Could you check a few things on this model? Use its own coordinates, in mm. Round coordinates to 2 decimals unless told otherwise and drop trailing zeros. Write each loop counter-clockwise with the first axis right and the second up, starting at its lowest first coordinate (ties: lowest second). Pieces come first, ordered by that corner, then holes. Notation, with made-up numbers: (32, -31) -> (49, -31) arc R18 cw to (49, -5) -> close; hole circle Ø8 at (18, 12). An arc over 180 degrees is marked (long way). Answer in a Markdown table with one row per item.
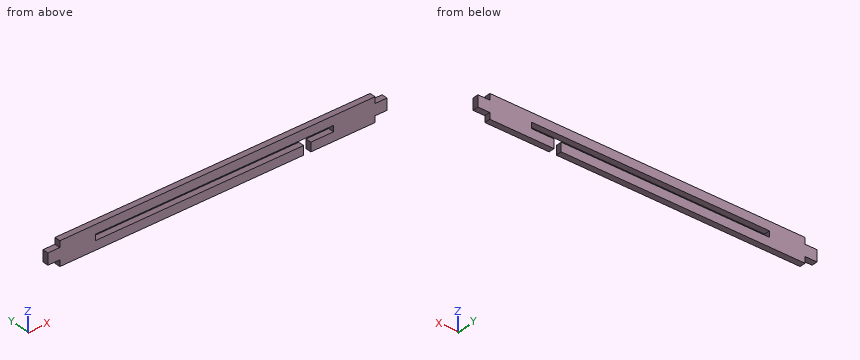
Autodesk Fusion 360 part; units mm, degrees
sketch "Sketch1" plane through (0, 0, 0) normal (0, 1, 0) x (1, 0, 0)
  line L0 (0, 0) -> (-265, 0)
  line L1 (-265, 0) -> (-265, -20)
  line L2 (-265, -20) -> (0, -20)
  line L3 (0, -20) -> (0, 0)
  dimension "d1" = 265
  dimension "d2" = 20
extrude "Extrude1" add sketch "Sketch1" along normal blind 5
sketch "Sketch3" plane through (0, 0, 0) normal (0, 1, 0) x (1, 0, 0)
  line L0 (-235, -7.5) -> (-35, -7.5)
  line L1 (-35, -7.5) -> (-35, -12.5)
  line L2 (-35, -12.5) -> (-235, -12.5)
  line L3 (-235, -12.5) -> (-235, -7.5)
  line L4 (0, 0) -> (-265, 0)
  line L5 (0, -20) -> (0, 0)
  dimension "d9" = 200
  dimension "d10" = 5
extrude "Extrude2" cut sketch "Sketch3" along normal blind 5
sketch "Sketch4" plane through (0, 0, 0) normal (0, 1, 0) x (1, 0, 0)
  line L0 (0, -5.25) -> (5, -5.25)
  line L1 (5, -5.25) -> (5, -14.75)
  line L2 (5, -14.75) -> (0, -14.75)
  line L3 (0, -14.75) -> (0, -5.25)
  line L4 (0, -20) -> (0, 0)
  dimension "d13" = 5
  dimension "d14" = 9.5
extrude "Extrude3" add sketch "Sketch4" along normal blind 5
sketch "Sketch5" plane through (-265, 0, 0) normal (-1, 0, 0) x (0, 0, 1)
  line L0 (0, 0) -> (20, 0)
  line L1 (20, 0) -> (20, 5)
  line L2 (20, 5) -> (0, 5)
  line L3 (0, 5) -> (0, 0)
sketch "Sketch6" plane through (0, 0, 0) normal (0, 1, 0) x (1, 0, 0)
  line L0 (-265, -5.25) -> (-270, -5.25)
  line L1 (-270, -5.25) -> (-270, -14.75)
  line L2 (-270, -14.75) -> (-265, -14.75)
  line L3 (-265, -14.75) -> (-265, -5.25)
  line L4 (-265, 0) -> (-265, -20)
  line L5 (-265, -20) -> (-265, 0)
  dimension "d17" = 9.5
  dimension "d18" = 5
extrude "Extrude4" add sketch "Sketch6" along normal blind 5
sketch "Sketch7" plane through (0, 0, 0) normal (0, 1, 0) x (1, 0, 0)
  line L0 (-60, 0) -> (-54, 0)
  line L1 (-54, 0) -> (-54, -7.5)
  line L2 (-54, -7.5) -> (-60, -7.5)
  line L3 (-60, -7.5) -> (-60, 0)
  line L4 (0, 0) -> (-265, 0)
  dimension "d21" = 6
  dimension "d22" = 7.5
extrude "Extrude5" cut sketch "Sketch7" along normal blind 5
sketch "Sketch8" plane through (0, 0, 0) normal (0, 1, 0) x (1, 0, 0)
  line L0 (5, -5.25) -> (10, -5.25)
  line L1 (10, -5.25) -> (10, -14.75)
  line L2 (10, -14.75) -> (5, -14.75)
  line L3 (5, -14.75) -> (5, -5.25)
  point P0 (5, -5.25)
  dimension "d25" = 9.5
extrude "Extrude6" add sketch "Sketch8" along normal blind 5
sketch "Sketch9" plane through (0, 0, 0) normal (0, 1, 0) x (1, 0, 0)
  line L0 (-270, -5.25) -> (-275, -5.25)
  line L1 (-275, -5.25) -> (-275, -14.75)
  line L2 (-275, -14.75) -> (-270, -14.75)
  line L3 (-270, -14.75) -> (-270, -5.25)
  point P0 (-270, -5.25)
  dimension "d28" = 5
  dimension "d29" = 9.5
extrude "Extrude7" add sketch "Sketch9" along normal blind 5
1) Imagine slicing it at A-A, the plane x = -135. Please give me the cut outline in (y, z), plus the area to 3 significant figures.
Findings:
| item | result |
|---|---|
| outline | (0, 0) -> (5, 0) -> (5, 7.5) -> (0, 7.5) -> close; (0, 12.5) -> (5, 12.5) -> (5, 20) -> (0, 20) -> close |
| area | 75.0 mm^2 |
2) Please list where these lines run through material, in increasing order: line 1 (X direction, y = 3.45, z = 8.75); line 2 (Z direction, x = -150, y = 2); line 3 (X direction, y = 0.8, z = 3.75).
Findings:
| item | result |
|---|---|
| line 1 | x = -275 to -235, -35 to 10 |
| line 2 | z = 0 to 7.5, 12.5 to 20 |
| line 3 | x = -265 to -60, -54 to 0 |
3) Imagine slicing it at B-B, the plane y = 2.8. Please give me the cut outline in (x, z).
Findings:
| item | result |
|---|---|
| outline | (-275, 5.25) -> (-265, 5.25) -> (-265, 0) -> (-60, 0) -> (-60, 7.5) -> (-235, 7.5) -> (-235, 12.5) -> (-35, 12.5) -> (-35, 7.5) -> (-54, 7.5) -> (-54, 0) -> (0, 0) -> (0, 5.25) -> (10, 5.25) -> (10, 14.75) -> (0, 14.75) -> (0, 20) -> (-265, 20) -> (-265, 14.75) -> (-275, 14.75) -> close |
4) For pin 1 (2.5 mm diameter, centred on x = 3, y = 3.5, fed in from -Z); pin 2 (2.5 mm diameter, centred on y = 2.5, z = 18.5, fed in from -X); pin 3 (10 mm diameter, centred on x = -189.5, z = 11, fed in from +Y); pin 4 (1.5 mm diameter, centred on y = 1.5, z = 1.5, fed in from +X), each with a flat end and sliding along its axis, tell me the tip position at first contact or that it passes through.
Findings:
| item | result |
|---|---|
| pin 1 | stops at z = 5.25 |
| pin 2 | stops at x = -265 |
| pin 3 | stops at y = 5 |
| pin 4 | stops at x = 0 |
5) Imagine slicing it at C-C, the plane z = 17.25. Please give me the cut outline in (x, y).
Findings:
| item | result |
|---|---|
| outline | (-265, 0) -> (0, 0) -> (0, 5) -> (-265, 5) -> close |
